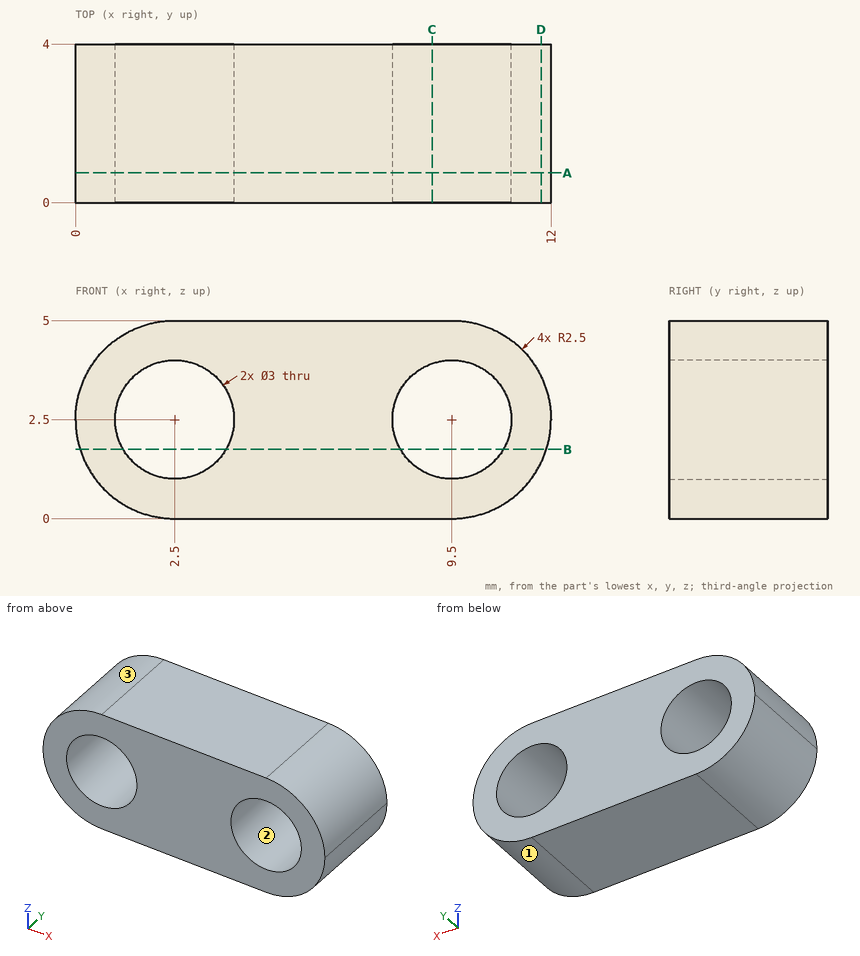
Input: dimensioned drawing with shaded views. Units: mm. Origin: part minimum x, y, z. Give positions to 0.01 mm unless a question says otherwise; leave off trailing zeros. Write each loop counter-clockwise with the first axis right and the second up, starting at its lowest first coordinate (ties: lowest second). Pieces come first, ordered by that corner, then holes.
1. Pull-direction query (Z, two-part tool) for the marked faces 1, 2 and 3; classes: +Z half, -Z half, draft (parallel to the pull), parting line (faces both ways), or undercut.
2. Section query D-D (x = 11.75). Return the cut outline in (y, z).
3. First-contact query: pin 1 (1.8 mm diameter, centred on x = 2.5, z = 2.5, fed in from -Y). Flat tip, straight axial feed; report the tip coordinate or a pass-through.
4. Material intervals for line 1 along X through (y, z) = (2.95, 2.5); line 2 along X through (y, z) = (0.85, 1.65); line 3 along Z through (x, y) = (8.25, 0.75), sorted ascending.
5. Section query A-A (y = 0.75). Count the separate pieces of the cut face and the enclosed holes in it, then the cut area to 3 significant figures.
6. Section query C-C (x = 9). Return the cut outline in (y, z).
7. Section query B-B (z = 1.75). Return the cut outline in (x, y) (3 decimals).
Output values:
1. face 1: -Z half
1. face 2: undercut
1. face 3: +Z half
2. outline: (0, 1.41) - (4, 1.41) - (4, 3.59) - (0, 3.59) - close
3. pin 1: passes through
4. line 1: x = 0 to 1, 4 to 8, 11 to 12
4. line 2: x = 0.15 to 1.26, 3.74 to 8.26, 10.74 to 11.85
4. line 3: z = 0 to 1.67, 3.33 to 5
5. separate pieces: 1
5. enclosed holes: 2
5. area: 40.5 mm2
6. outline: (0, 0) - (4, 0) - (4, 1.09) - (0, 1.09) - close; (0, 3.91) - (4, 3.91) - (4, 5) - (0, 5) - close
7. outline: (0.115, 0) - (1.201, 0) - (1.201, 4) - (0.115, 4) - close; (3.799, 0) - (8.201, 0) - (8.201, 4) - (3.799, 4) - close; (10.799, 0) - (11.885, 0) - (11.885, 4) - (10.799, 4) - close
